```python
from build123d import *

# Parameters (mm, degrees)
SKETCH1_R           = 3
BOSS_EXTRUDE1_DEPTH = 5


with BuildPart() as part:
    # Sketch1 → Boss-Extrude1 (new body)
    with BuildSketch(Plane.XY):
        with BuildLine():
            add(Edge.make_bspline(
                [(0, 30), (3.243669136, 29.514932873), (1.18511812, 25.21974269), (3.910973785, 24.69291666)],
                knots=[0, 0, 0, 0, 0.984502581, 0.984502581, 0.984502581, 0.984502581], degree=3))
            add(Edge.make_bspline(
                [(0, 30), (-3.243669136, 29.514932873), (-1.18511812, 25.21974269), (-3.910973785, 24.69291666)],
                knots=[0, 0, 0, 0, 0.984502581, 0.984502581, 0.984502581, 0.984502581], degree=3))
            add(Edge.make_bspline(
                [(-9.270509831, 28.531695489), (-6.035703177, 29.072718124), (-6.666214775, 24.351622264), (-3.910973785, 24.69291666)],
                knots=[0, 0, 0, 0, 0.984502581, 0.984502581, 0.984502581, 0.984502581], degree=3))
            add(Edge.make_bspline(
                [(-9.270509831, 28.531695489), (-12.205528514, 27.06802035), (-8.920443395, 23.619178985), (-11.350087992, 22.275801932)],
                knots=[0, 0, 0, 0, 0.984502581, 0.984502581, 0.984502581, 0.984502581], degree=3))
            add(Edge.make_bspline(
                [(-17.633557569, 24.270509831), (-14.72425881, 25.784663164), (-13.865012121, 21.099795383), (-11.350087992, 22.275801932)],
                knots=[0, 0, 0, 0, 0.984502581, 0.984502581, 0.984502581, 0.984502581], degree=3))
            add(Edge.make_bspline(
                [(-17.633557569, 24.270509831), (-19.972625721, 21.971501401), (-15.782573519, 19.706605477), (-17.678176506, 17.678176506)],
                knots=[0, 0, 0, 0, 0.984502581, 0.984502581, 0.984502581, 0.984502581], degree=3))
            add(Edge.make_bspline(
                [(-24.270509831, 17.633557569), (-21.971501401, 19.972625721), (-19.706605477, 15.782573519), (-17.678176506, 17.678176506)],
                knots=[0, 0, 0, 0, 0.984502581, 0.984502581, 0.984502581, 0.984502581], degree=3))
            add(Edge.make_bspline(
                [(-24.270509831, 17.633557569), (-25.784663164, 14.72425881), (-21.099795383, 13.865012121), (-22.275801932, 11.350087992)],
                knots=[0, 0, 0, 0, 0.984502581, 0.984502581, 0.984502581, 0.984502581], degree=3))
            add(Edge.make_bspline(
                [(-28.531695489, 9.270509831), (-27.06802035, 12.205528514), (-23.619178985, 8.920443395), (-22.275801932, 11.350087992)],
                knots=[0, 0, 0, 0, 0.984502581, 0.984502581, 0.984502581, 0.984502581], degree=3))
            add(Edge.make_bspline(
                [(-28.531695489, 9.270509831), (-29.072718124, 6.035703177), (-24.351622264, 6.666214775), (-24.69291666, 3.910973785)],
                knots=[0, 0, 0, 0, 0.984502581, 0.984502581, 0.984502581, 0.984502581], degree=3))
            add(Edge.make_bspline(
                [(-30, 0), (-29.514932873, 3.243669136), (-25.21974269, 1.18511812), (-24.69291666, 3.910973785)],
                knots=[0, 0, 0, 0, 0.984502581, 0.984502581, 0.984502581, 0.984502581], degree=3))
            add(Edge.make_bspline(
                [(-30, 0), (-29.514932873, -3.243669136), (-25.21974269, -1.18511812), (-24.69291666, -3.910973785)],
                knots=[0, 0, 0, 0, 0.984502581, 0.984502581, 0.984502581, 0.984502581], degree=3))
            add(Edge.make_bspline(
                [(-28.531695489, -9.270509831), (-29.072718124, -6.035703177), (-24.351622264, -6.666214775), (-24.69291666, -3.910973785)],
                knots=[0, 0, 0, 0, 0.984502581, 0.984502581, 0.984502581, 0.984502581], degree=3))
            add(Edge.make_bspline(
                [(-28.531695489, -9.270509831), (-27.06802035, -12.205528514), (-23.619178985, -8.920443395), (-22.275801932, -11.350087992)],
                knots=[0, 0, 0, 0, 0.984502581, 0.984502581, 0.984502581, 0.984502581], degree=3))
            add(Edge.make_bspline(
                [(-24.270509831, -17.633557569), (-25.784663164, -14.72425881), (-21.099795383, -13.865012121), (-22.275801932, -11.350087992)],
                knots=[0, 0, 0, 0, 0.984502581, 0.984502581, 0.984502581, 0.984502581], degree=3))
            add(Edge.make_bspline(
                [(-24.270509831, -17.633557569), (-21.971501401, -19.972625721), (-19.706605477, -15.782573519), (-17.678176506, -17.678176506)],
                knots=[0, 0, 0, 0, 0.984502581, 0.984502581, 0.984502581, 0.984502581], degree=3))
            add(Edge.make_bspline(
                [(-17.633557569, -24.270509831), (-19.972625721, -21.971501401), (-15.782573519, -19.706605477), (-17.678176506, -17.678176506)],
                knots=[0, 0, 0, 0, 0.984502581, 0.984502581, 0.984502581, 0.984502581], degree=3))
            add(Edge.make_bspline(
                [(-17.633557569, -24.270509831), (-14.72425881, -25.784663164), (-13.865012121, -21.099795383), (-11.350087992, -22.275801932)],
                knots=[0, 0, 0, 0, 0.984502581, 0.984502581, 0.984502581, 0.984502581], degree=3))
            add(Edge.make_bspline(
                [(-9.270509831, -28.531695489), (-12.205528514, -27.06802035), (-8.920443395, -23.619178985), (-11.350087992, -22.275801932)],
                knots=[0, 0, 0, 0, 0.984502581, 0.984502581, 0.984502581, 0.984502581], degree=3))
            add(Edge.make_bspline(
                [(-9.270509831, -28.531695489), (-6.035703177, -29.072718124), (-6.666214775, -24.351622264), (-3.910973785, -24.69291666)],
                knots=[0, 0, 0, 0, 0.984502581, 0.984502581, 0.984502581, 0.984502581], degree=3))
            add(Edge.make_bspline(
                [(0, -30), (-3.243669136, -29.514932873), (-1.18511812, -25.21974269), (-3.910973785, -24.69291666)],
                knots=[0, 0, 0, 0, 0.984502581, 0.984502581, 0.984502581, 0.984502581], degree=3))
            add(Edge.make_bspline(
                [(0, -30), (3.243669136, -29.514932873), (1.18511812, -25.21974269), (3.910973785, -24.69291666)],
                knots=[0, 0, 0, 0, 0.984502581, 0.984502581, 0.984502581, 0.984502581], degree=3))
            add(Edge.make_bspline(
                [(9.270509831, -28.531695489), (6.035703177, -29.072718124), (6.666214775, -24.351622264), (3.910973785, -24.69291666)],
                knots=[0, 0, 0, 0, 0.984502581, 0.984502581, 0.984502581, 0.984502581], degree=3))
            add(Edge.make_bspline(
                [(9.270509831, -28.531695489), (12.205528514, -27.06802035), (8.920443395, -23.619178985), (11.350087992, -22.275801932)],
                knots=[0, 0, 0, 0, 0.984502581, 0.984502581, 0.984502581, 0.984502581], degree=3))
            add(Edge.make_bspline(
                [(17.633557569, -24.270509831), (14.72425881, -25.784663164), (13.865012121, -21.099795383), (11.350087992, -22.275801932)],
                knots=[0, 0, 0, 0, 0.984502581, 0.984502581, 0.984502581, 0.984502581], degree=3))
            add(Edge.make_bspline(
                [(17.633557569, -24.270509831), (19.972625721, -21.971501401), (15.782573519, -19.706605477), (17.678176506, -17.678176506)],
                knots=[0, 0, 0, 0, 0.984502581, 0.984502581, 0.984502581, 0.984502581], degree=3))
            add(Edge.make_bspline(
                [(24.270509831, -17.633557569), (21.971501401, -19.972625721), (19.706605477, -15.782573519), (17.678176506, -17.678176506)],
                knots=[0, 0, 0, 0, 0.984502581, 0.984502581, 0.984502581, 0.984502581], degree=3))
            add(Edge.make_bspline(
                [(24.270509831, -17.633557569), (25.784663164, -14.72425881), (21.099795383, -13.865012121), (22.275801932, -11.350087992)],
                knots=[0, 0, 0, 0, 0.984502581, 0.984502581, 0.984502581, 0.984502581], degree=3))
            add(Edge.make_bspline(
                [(28.531695489, -9.270509831), (27.06802035, -12.205528514), (23.619178985, -8.920443395), (22.275801932, -11.350087992)],
                knots=[0, 0, 0, 0, 0.984502581, 0.984502581, 0.984502581, 0.984502581], degree=3))
            add(Edge.make_bspline(
                [(28.531695489, -9.270509831), (29.072718124, -6.035703177), (24.351622264, -6.666214775), (24.69291666, -3.910973785)],
                knots=[0, 0, 0, 0, 0.984502581, 0.984502581, 0.984502581, 0.984502581], degree=3))
            add(Edge.make_bspline(
                [(30, 0), (29.514932873, -3.243669136), (25.21974269, -1.18511812), (24.69291666, -3.910973785)],
                knots=[0, 0, 0, 0, 0.984502581, 0.984502581, 0.984502581, 0.984502581], degree=3))
            add(Edge.make_bspline(
                [(30, 0), (29.514932873, 3.243669136), (25.21974269, 1.18511812), (24.69291666, 3.910973785)],
                knots=[0, 0, 0, 0, 0.984502581, 0.984502581, 0.984502581, 0.984502581], degree=3))
            add(Edge.make_bspline(
                [(28.531695489, 9.270509831), (29.072718124, 6.035703177), (24.351622264, 6.666214775), (24.69291666, 3.910973785)],
                knots=[0, 0, 0, 0, 0.984502581, 0.984502581, 0.984502581, 0.984502581], degree=3))
            add(Edge.make_bspline(
                [(28.531695489, 9.270509831), (27.06802035, 12.205528514), (23.619178985, 8.920443395), (22.275801932, 11.350087992)],
                knots=[0, 0, 0, 0, 0.984502581, 0.984502581, 0.984502581, 0.984502581], degree=3))
            add(Edge.make_bspline(
                [(24.270509831, 17.633557569), (25.784663164, 14.72425881), (21.099795383, 13.865012121), (22.275801932, 11.350087992)],
                knots=[0, 0, 0, 0, 0.984502581, 0.984502581, 0.984502581, 0.984502581], degree=3))
            add(Edge.make_bspline(
                [(24.270509831, 17.633557569), (21.971501401, 19.972625721), (19.706605477, 15.782573519), (17.678176506, 17.678176506)],
                knots=[0, 0, 0, 0, 0.984502581, 0.984502581, 0.984502581, 0.984502581], degree=3))
            add(Edge.make_bspline(
                [(17.633557569, 24.270509831), (19.972625721, 21.971501401), (15.782573519, 19.706605477), (17.678176506, 17.678176506)],
                knots=[0, 0, 0, 0, 0.984502581, 0.984502581, 0.984502581, 0.984502581], degree=3))
            add(Edge.make_bspline(
                [(17.633557569, 24.270509831), (14.72425881, 25.784663164), (13.865012121, 21.099795383), (11.350087992, 22.275801932)],
                knots=[0, 0, 0, 0, 0.984502581, 0.984502581, 0.984502581, 0.984502581], degree=3))
            add(Edge.make_bspline(
                [(9.270509831, 28.531695489), (12.205528514, 27.06802035), (8.920443395, 23.619178985), (11.350087992, 22.275801932)],
                knots=[0, 0, 0, 0, 0.984502581, 0.984502581, 0.984502581, 0.984502581], degree=3))
            add(Edge.make_bspline(
                [(9.270509831, 28.531695489), (6.035703177, 29.072718124), (6.666214775, 24.351622264), (3.910973785, 24.69291666)],
                knots=[0, 0, 0, 0, 0.984502581, 0.984502581, 0.984502581, 0.984502581], degree=3))
        make_face()
        Circle(SKETCH1_R, mode=Mode.SUBTRACT)
    extrude(amount=BOSS_EXTRUDE1_DEPTH)


solid = part.part
```
Could you check a few things on this model? Use its own coordinates, in mm. Coordinates: 2 decimals unless noted, no trailing zeros. Use one line per item in the form item = value. Start each with the question number.
1. We'd pull the mould along Y, two halves only. Please class faces 1 (the cylindrical face through (-3, 0, 2)), 2 (the flat face through (0, -6, 5)): +Y half, -Y half, draft (parallel to the pull), parting line (faces both ways), or undercut.
2. For pin 1 (9.5 mm diameter, centred on x = 0, y = 0, fed in from +Z); pin 2 (1 mm diameter, centred on x = -15, z = 2, fed in from -Y); pin 3 (3 mm diameter, centred on y = -11.5, z = 1, fed in from -X); pin 4 (3 mm diameter, centred on x = 11.5, z = 0.5, fed in from +Y), each with a flat end and sliding along its axis, tell me the tip position at first contact or that it passes through.
3. Please list where these lines run through material, in increasing order: line 1 (Y direction, x = 0, z = 3.35); line 2 (X direction, y = 27, z = 3.3); line 3 (X direction, y = -18, z = 4.4).
Geometry says:
q1.face_1 = undercut
q1.face_2 = draft
q2.pin_1 = 5
q2.pin_2 = -24.3
q2.pin_3 = -28.01
q2.pin_4 = 28.01
q3.line_1 = -30 to -3, 3 to 30
q3.line_2 = -10.52 to -6.59, -2.22 to 2.22, 6.59 to 10.52
q3.line_3 = -23.84 to -21.26, -17.43 to 17.43, 21.26 to 23.84
